Design review of the part built by this model. Coordinates are the model's own, in mm. Face numbers are marked on the shaded views. A direction names the side the tool comes from. Give positions to 0.01 mm unless a question says otherwise; leave off trailing zeros. Order: outer loops, then holes, each group sorted by start corner. A loop starts at its lowest first (then second) coordinate and runs counter-clockwise, first axis right, second up. Notation, with made-up numbers: M 55.5,51.25 L 71.5,51.25 A22 cw 71.5,83.25 Z; hole C -22.5,-9 d8. An arc over 180 degrees is marked long. Answer as a JSON object with one key per item and string values.
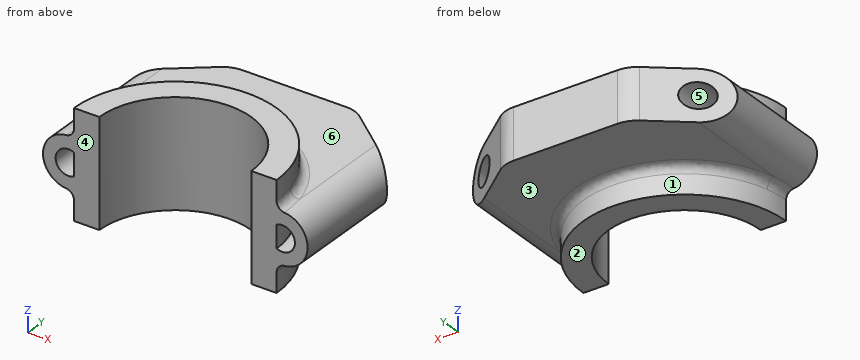
from build123d import *

# Parameters (mm, degrees)
BOSS_EXTRUDE1_DEPTH = 38
SKETCH3_R           = 4.5
BOSS_EXTRUDE2_DEPTH = 60
CUT_EXTRUDE1_DEPTH  = 60
CUT_EXTRUDE2_DEPTH  = 60
FILLET1_R           = 10
FILLET2_R           = 3


with BuildPart() as part:
    # Sketch2 → Boss-Extrude1 (new body)
    with BuildSketch(Plane.XY):
        with BuildLine():
            Line((-36, 0), (-27, 0))
            ThreePointArc((-27, 0), (0, 27), (27, 0))
            Line((27, 0), (36, 0))
            ThreePointArc((36, 0), (0, 36), (-36, 0))
        make_face()
    extrude(amount=BOSS_EXTRUDE1_DEPTH)

    # Sketch3 → Boss-Extrude2 (add)
    with BuildSketch(Plane(origin=(0, 60, 0), x_dir=(-1, 0, 0), z_dir=(0, -1, 0))):
        with BuildLine():
            Line((38, -28), (-38, -28))
            ThreePointArc((-38, -28), (-47, -19), (-38, -10))
            Line((-38, -10), (38, -10))
            ThreePointArc((38, -10), (47, -19), (38, -28))
        make_face()
        with Locations((38, -19)):
            Circle(SKETCH3_R, mode=Mode.SUBTRACT)
        with Locations((-38, -19)):
            Circle(SKETCH3_R, mode=Mode.SUBTRACT)
    extrude(amount=BOSS_EXTRUDE2_DEPTH)

    # Sketch4 → Cut-Extrude1 (cut)
    with BuildSketch(Plane.XY.offset(28)):
        with BuildLine():
            Line((-27, 0), (27, 0))
            ThreePointArc((27, 0), (0, 27), (-27, 0))
        make_face()
    extrude(amount=-CUT_EXTRUDE1_DEPTH, mode=Mode.SUBTRACT)

    # Sketch5 → Cut-Extrude2 (cut)
    with BuildSketch(Plane.XY.offset(28)):
        Polygon((-47, 40), (-22, 60), (-47, 60), align=None)
        Polygon((47, 40), (22, 60), (47, 60), align=None)
    extrude(amount=-CUT_EXTRUDE2_DEPTH, mode=Mode.SUBTRACT)

    # Fillet1
    fillet1_edges = [part.edges().sort_by_distance(p)[0] for p in [
        (-22, 60, 19),
        (22, 60, 19),
    ]]
    fillet(fillet1_edges, radius=FILLET1_R)

    # Fillet2
    fillet2_edges = [part.edges().sort_by_distance(p)[0] for p in [
        (0, 36, 10),
        (0, 36, 28),
    ]]
    fillet(fillet2_edges, radius=FILLET2_R)


solid = part.part
(1) We need section A-A (z = 19). Write out the cut boundary in (x, y).
Checked values:
{"outline": "M -47,0 L -42.5,0 L -42.5,43.6 L -47,40 Z; M -36,0 L -27,0 A27 cw 27,0 L 36,0 A36 ccw 33.5,13.18 L 33.5,50.8 L 24.74,57.81 A10 ccw 18.49,60 L -18.49,60 A10 ccw -24.74,57.81 L -33.5,50.8 L -33.5,13.18 A36 ccw Z; M 42.5,0 L 47,0 L 47,40 L 42.5,43.6 Z"}
(2) Tool access review of the marked faces 1 and 2: name each direction out of +Z, -Z, +X, -X, +Y, -Y from which nothing blocks a thin tool from reaching the whole face with its end or side.
Checked values:
{"face 1": "-Z, +Y", "face 2": "-Z, +X, -X, +Y, -Y"}
(3) We need section B-B (y = 6). Count the separate pieces of the cut face and the enclosed holes in it, plus the area to 3 significant figures.
Checked values:
{"separate pieces": "2", "enclosed holes": "2", "area": "943 mm^2"}
(4) We need section C-C (z = 13.5). Write out the cut boundary in (x, y).
Checked values:
{"outline": "M -45.12,0 L -27,0 A27 cw 27,0 L 45.12,0 L 45.12,41.5 L 24.74,57.81 A10 ccw 18.49,60 L -18.49,60 A10 ccw -24.74,57.81 L -45.12,41.5 Z"}
(5) Draft analysis for pull direction Z (two halves, no side actions). For the marked faces 3, 4, 5 and 6, state which applies: +Z half, -Z half, draft (parallel to the pull), parting line (faces both ways), or undercut.
Checked values:
{"face 3": "-Z half", "face 4": "draft", "face 5": "undercut", "face 6": "+Z half"}
(6) To check wall thickness, follow L1, parallel to X at y = 35, z = 19; L2, parallel to X at y = 16, z = 19; L3, parallel to Z at x = -38, y = 31. State the ranges of each line that lie inside material, in increasing order. Write a range as from..to.
Checked values:
{"L1": "x = -47..-42.5, -33.5..33.5, 42.5..47", "L2": "x = -47..-42.5, -33.5..-21.75, 21.75..33.5, 42.5..47", "L3": "z = 10..14.5, 23.5..28"}
(7) Insertion check: pin 1 (4 mm diameter, centred on x = 34.5, z = 23, fed in from +Y); pin 2 (3 mm diameter, centred on x = -32, z = 9.5, fed in from +Y); pin 3 (5 mm diameter, centred on x = -29, z = 23, fed in from +Y). Each pin has a flat end and moves straight along its axis. Give the tip position at first contact, or say it passes through.
Checked values:
{"pin 1": "stops at y = 51.6", "pin 2": "stops at y = 53.13", "pin 3": "stops at y = 56.4"}
